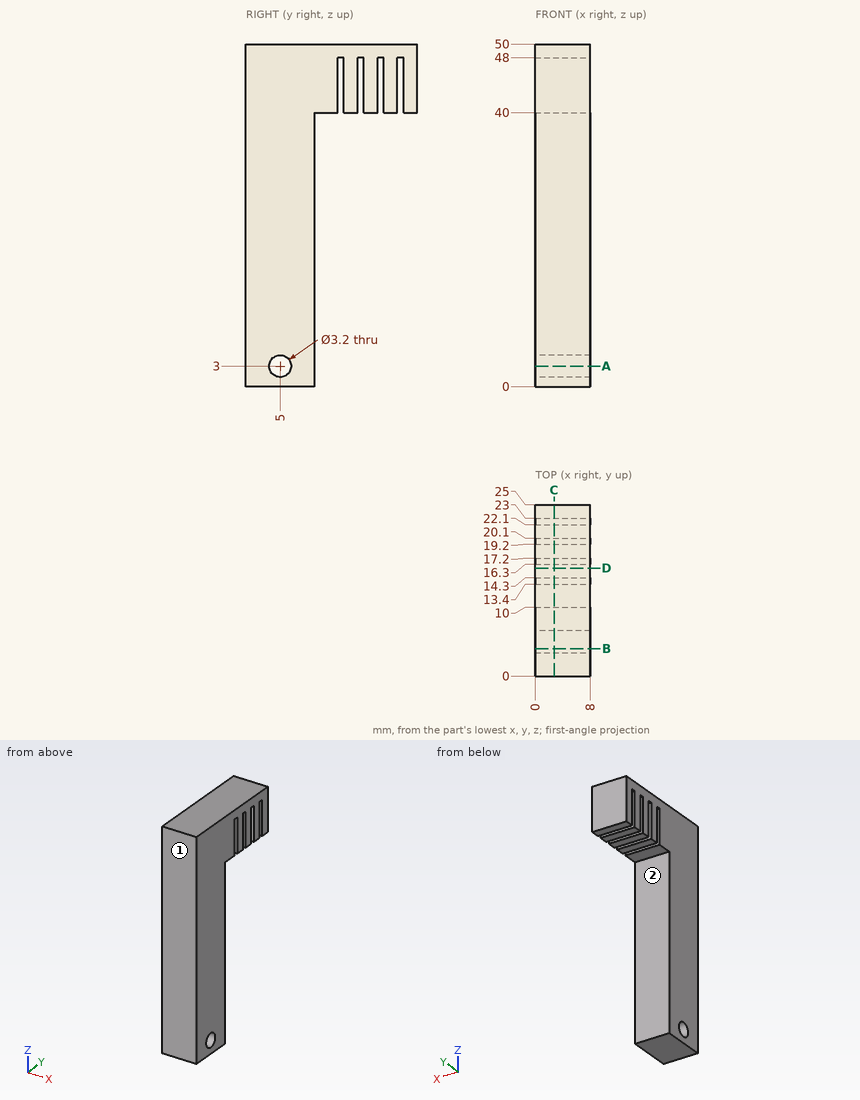
Can you work these out from the drawing? Everything is in mm from the part's minimum corner. A direction names the side the tool comes from. Round coordinates to 2 decimals unless told otherwise and drop trailing zeros. Loops run counter-clockwise (first coordinate to the right, second up) from the corner with the lowest first, then second, coordinate; pieces in that order, holes last. Notation, with made-up numbers: (0.5, 82) - (58.5, 82) arc R26 ccw to (58.5, 116) - close; hole circle Ø9 at (53.5, 87.25). An arc over 180 degrees is marked (long way). Write item = value, one per line. Start each with the question number.
(1) If we section it at D-D (y = 15.75): Please give me the cut outline in (x, z), and give its area (3 significant figures).
(2) For P1, Ø0.6, axis at x = 3.5, y = 23.5, coming from the -Z side; P2, Ø4, axis at y = 11, z = 31.5, coming from the -X side; P3, Ø2, axis at x = 7, z = 26.5, coming from the +Y side, each with a flat end and sliding along its axis, tell me the tip position at first contact or that it passes through.
(3) If I drill on probe 1 along Y at (x, z) = (4.25, 47); probe 2 along Z at (x, y) = (4.75, 5); probe 3 along Z at (x, y) = (0.5, 12.75), over which ranges is the centre line in solid material (lowest first)? Write a range as [from, to].
(4) For the marked faces 1 and 2, which set-ups out of +Z, -Z, +X, -X, +Y, -Y let a thin tool reach every point of the face, with its end or its side?
(5) If we section it at B-B (y = 4): Please give me the cut outline in (x, z).
(6) If we section it at C-C (x = 2.75): Please give me the cut outline in (y, z), and give its area (3 significant figures).
(7) If we section it at A-A (z = 3): Please give me the cut outline in (x, y).
Ans:
q1.outline = (0, 40) - (8, 40) - (8, 50) - (0, 50) - close
q1.area = 80.0 mm²
q2.P1 = 40
q2.P2 = 0
q2.P3 = 10
q3.probe_1 = [0, 13.4], [14.3, 16.3], [17.2, 19.2], [20.1, 22.1], [23, 25]
q3.probe_2 = [0, 1.4], [4.6, 50]
q3.probe_3 = [40, 50]
q4.face_1 = +Z, -Z, +X, -X, -Y
q4.face_2 = -Z, +X, -X, +Y
q5.outline = (0, 0) - (8, 0) - (8, 1.75) - (0, 1.75) - close; (0, 4.25) - (8, 4.25) - (8, 50) - (0, 50) - close
q6.outline = (0, 0) - (10, 0) - (10, 40) - (13.4, 40) - (13.4, 48) - (14.3, 48) - (14.3, 40) - (16.3, 40) - (16.3, 48) - (17.2, 48) - (17.2, 40) - (19.2, 40) - (19.2, 48) - (20.1, 48) - (20.1, 40) - (22.1, 40) - (22.1, 48) - (23, 48) - (23, 40) - (25, 40) - (25, 50) - (0, 50) - close; hole circle Ø3.2 at (5, 3)
q6.area = 613 mm²
q7.outline = (0, 0) - (8, 0) - (8, 3.4) - (0, 3.4) - close; (0, 6.6) - (8, 6.6) - (8, 10) - (0, 10) - close
